```python
from build123d import *

# Parameters (mm, degrees)
F2_R     = 26
F3_DEPTH = 40
F4_R     = 24.5
F5_DEPTH = 5
F6_R     = 26
F7_DEPTH = 9
F8_R     = 3.5
F9_DEPTH = 54.001


with BuildPart() as f1:
    # F0 (on Front) → F1 (revolve)
    with BuildSketch(Plane.XZ):
        with BuildLine():
            Line((31, 53.175), (22.9837517073, 53.175))
            ThreePointArc((22.9837517073, 53.175), (20.3059838669, 51.7059262565), (20.1062244835, 48.658187019))
            Line((20.1062244835, 48.658187019), (25.4609225305, 37.175))
            Line((25.4609225305, 37.175), (-23, 37.175))
            Line((-23, 37.175), (-23, -1.8250067694))
            Line((-23, -1.8250067694), (31, -1.8250067694))
            Line((31, -1.8250067694), (31, 37.175))
            Line((31, 37.175), (31, 53.175))
        make_face()
    revolve(axis=Axis((4, 0, -1.8250067694), (-1, 0, 0)))

    # F2 (on face) → F3 (cut)
    with BuildSketch(Plane.YZ.offset(31)):
        with Locations((0, -1.8250067694)):
            Circle(F2_R)
    extrude(amount=-F3_DEPTH, mode=Mode.SUBTRACT)

    # F4 (on face) → F5 (cut)
    with BuildSketch(Plane.YZ.offset(-9)):
        with Locations((0, -1.8250067694)):
            Circle(F4_R)
    extrude(amount=-F5_DEPTH, mode=Mode.SUBTRACT)

    # F6 (on face) → F7 (cut)
    with BuildSketch(Plane(origin=(-23, 0, 0), x_dir=(0, -1, 0), z_dir=(-1, 0, 0))):
        with Locations((0, -1.8250067694)):
            Circle(F6_R)
    extrude(amount=-F7_DEPTH, mode=Mode.SUBTRACT)

    # F8 (on face) → F9 (cut, through all)
    with BuildSketch(Plane(origin=(-23, 0, 0), x_dir=(0, -1, 0), z_dir=(-1, 0, 0))):
        with Locations((-29.0118510268, 14.9249932306)):
            Circle(F8_R)
        with Locations((-29.0118510268, -18.5750067694)):
            Circle(F8_R)
        with Locations((0, -35.3250067694)):
            Circle(F8_R)
        with Locations((29.0118510268, -18.5750067694)):
            Circle(F8_R)
        with Locations((29.0118510268, 14.9249932306)):
            Circle(F8_R)
        with BuildLine():
            Line((0, 31.6749932306), (0, 35.1749932306))
            ThreePointArc((0, 35.1749932306), (-3.5, 31.6749932306), (0, 28.1749932306))
            Line((0, 28.1749932306), (0, 31.6749932306))
        make_face()
        with BuildLine():
            ThreePointArc((0, 28.1749932306), (2.4748737342, 29.2001194964), (3.5, 31.6749932306))
            ThreePointArc((3.5, 31.6749932306), (2.4748737342, 34.1498669647), (0, 35.1749932306))
            Line((0, 35.1749932306), (0, 31.6749932306))
            Line((0, 31.6749932306), (0, 28.1749932306))
        make_face()
    extrude(amount=-F9_DEPTH, mode=Mode.SUBTRACT)


solid = f1.part
```
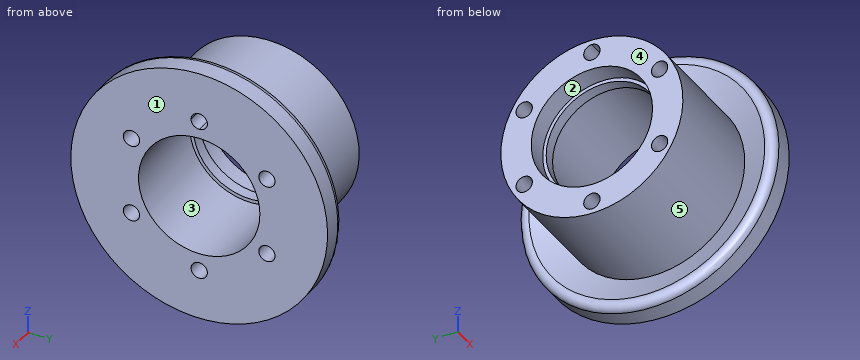
For this review, take the finished solid that the model builds, in its own axes (mm). Face numbers are marked on the shaded views. A direction names the side the tool comes from. Round coordinates to 2 decimals unless told otherwise and drop trailing zeros. Write each loop counter-clockwise with the first axis right and the second up, starting at its lowest first coordinate (ties: lowest second). Pieces come first, ordered by that corner, then holes. Notation, with made-up numbers: (-5, -29) -> (39, -29) arc R22 cw to (39, -6) -> close; hole circle Ø2 at (13.5, 8.25). An arc over 180 degrees is marked (long way). Use one line per item in the form item = value.
1) Mouldability with a two-part tool opening along Z and no side actions: class the marked faces 1 and 2 as +Z half, -Z half, draft (parallel to the pull), parting line (faces both ways), or undercut.
Found:
face_1 = draft
face_2 = undercut
2) Take a section at A-A, the plane x = -11. Write out the cut boundary in (y, z) (3 decimals), and give its area (3 significant figures).
Found:
outline = circle Ø78 at (0, -1.825); hole circle Ø7 at (-29.012, -18.575); hole circle Ø7 at (-29.012, 14.925); hole circle Ø49 at (0, -1.825); hole circle Ø7 at (0, -35.325); hole circle Ø7 at (0, 31.675); hole circle Ø7 at (29.012, -18.575); hole circle Ø7 at (29.012, 14.925)
area = 2,660 mm2
3) Take a section at B-B, the plane x = -1. Write out the cut boundary in (y, z) (3 decimals), and give its area (3 significant figures).
Found:
outline = circle Ø78 at (0, -1.825); hole circle Ø7 at (-29.012, -18.575); hole circle Ø7 at (-29.012, 14.925); hole circle Ø52 at (0, -1.825); hole circle Ø7 at (0, -35.325); hole circle Ø7 at (0, 31.675); hole circle Ø7 at (29.012, -18.575); hole circle Ø7 at (29.012, 14.925)
area = 2,420 mm2
4) Tool access review of the marked faces 3, 4 and 5: name each direction out of +Z, -Z, +X, -X, +Y, -Y from which nothing blocks a thin tool from reaching the whole face with its end or side.
Found:
face_3 = +X
face_4 = +Z, -Z, -X, +Y, -Y
face_5 = -X
5) To check wall thickness, follow L1, parallel to Z at x = 1, y = 1; L2, parallel to Y at x = -19.5, z = 12.5; L3, parallel to Y at x = -18, z = -21. State the ranges of each line that lie inside material, in increasing order. Write a range as from..to.
Found:
L1 = -40.81..-38.68, -31.97..-27.81, 24.16..28.32, 35.03..37.16
L2 = -36.27..-31.54, -26.49..-21.7, 21.7..26.49, 31.54..36.27
L3 = -33.96..-31.54, -26.49..-17.56, 17.56..26.49, 31.54..33.96
6) Clearance check with flat-ended pins moving along their axes: pin 1 (5.5 mm diameter, centred on y = 29.01, z = 14.92, fed in from -X); pin 2 (6 mm diameter, centred on x = 10, z = -21.5, fed in from -Y); pin 3 (1 mm diameter, centred on x = -15.5, z = 26, fed in from +Y); pin 4 (2 mm diameter, centred on x = -6.5, y = -26.5, fed in from -Z). State where each tip first meets the part, or that it passes through.
Found:
pin_1 = through
pin_2 = -35.26
pin_3 = 27.83
pin_4 = -31.33
